Geometry check sheet. Reference: the model listing, model coordinates, mm. A direction names the side the tool comes from. Round coordinates to 2 decimals unless told otherwise and drop trailing zeros. Order: outer loops, then holes, each group sorted by start corner. A loop starts at its lowest first (then second) coordinate and runs counter-clockwise, first axis right, second up.
(1) Set-up check for faces 1 (the face through (-19, 12, 11)), 2 (the face through (34.479, 8.248, 15.287)), 3 (the face through (-19, -9, 17)): record each of +Z, -Z, +X, -X, +Y, -Y from which the full face is reachable in a straight line by a thin tool's end or side.
(2) Sectioned sample at A-A (x = -1.5). Record the boundary of the cut face in (y, z).
(3) Sectioned sample at B-B (z = 7). Give the number of separate pieces and of enclosed holes in the cut face, plus the area to 3 significant figures.
(4) Go/stop test with flat-tipped pins: pin 1 (4 mm diameter, centred on x = 29.5, y = 11.5, fed in from -Z); pin 2 (2 mm diameter, centred on x = 35, z = 12.5, fed in from -Y). Record where each tip stops, or that it passes through.
(5) Material ranges on line 1 along X through (y, z) = (15.5, 7.75); line 2 along Y through (x, z) = (2, 6.5); line 3 along X through (y, z) = (1, 4), recorded low to high.
(6) Release check for a two-part mould opening along X. For faces 4 (the face through (35.287, 17.248, 9.86)), 5 (the face through (34.479, 8.287, 9.752)), 6 (the face through (-32.1, 14.14, 7.89)) record: +X half, -X half, draft (parallel to the pull), parting line (faces both ways), or undercut.
(7) Sectioned sample at C-C (y = 14). Record the boundary of the cut face in (x, z), plus the area to 3 significant figures.
(8) Sectioned sample at D-D (z = 16.75). Record the boundary of the cut face in (x, y).
from build123d import *

# Parameters (mm, degrees)
PAD_DEPTH            = 20
POCKET_DEPTH         = 16
SKETCH002_R          = 1.75
SKETCH002_W          = 28
SKETCH002_H          = 22
POCKET001_DEPTH      = 4
POCKET002_DEPTH      = 3
SKETCH004_W          = 27
SKETCH004_H          = 18
POCKET003_DEPTH      = 3
SKETCH005_R          = 1
POCKET004_DEPTH      = 10
SKETCH007_W          = 13
SKETCH007_H          = 11
PAD001_DEPTH         = 6
POCKET005_DEPTH      = 5
POCKET005_DEPTH_BACK = 10
SKETCH008_R          = 4
POCKET006_DEPTH      = 3
SKETCH009_R          = 3.5
POCKET007_DEPTH      = 3


with BuildPart() as part:
    # Sketch001 (on Sketch) → Pad (new body)
    with BuildSketch(Plane.XY):
        with BuildLine():
            Line((-33.5, 18), (33.5, 18))
            ThreePointArc((36, 15.5), (35.267767, 17.267767), (33.5, 18))
            Line((36, 15.5), (36, -15.5))
            ThreePointArc((33.5, -18), (35.267767, -17.267767), (36, -15.5))
            Line((33.5, -18), (-33.5, -18))
            ThreePointArc((-36, -15.5), (-35.267767, -17.267767), (-33.5, -18))
            Line((-36, -15.5), (-36, 15.5))
            ThreePointArc((-33.5, 18), (-35.267767, 17.267767), (-36, 15.5))
        make_face()
    extrude(amount=PAD_DEPTH)

    # Sketch → Pocket (cut)
    with BuildSketch(Plane.XY):
        with BuildLine():
            Line((-30, 15), (30, 15))
            ThreePointArc((33, 12), (32.12132, 14.12132), (30, 15))
            Line((33, 12), (33, -12))
            ThreePointArc((30, -15), (32.12132, -14.12132), (33, -12))
            Line((30, -15), (-30, -15))
            ThreePointArc((-33, -12), (-32.12132, -14.12132), (-30, -15))
            Line((-33, -12), (-33, 12))
            ThreePointArc((-30, 15), (-32.12132, 14.12132), (-33, 12))
        make_face()
    extrude(amount=POCKET_DEPTH, mode=Mode.SUBTRACT)

    # Sketch002 (on Sketch) → Pocket001 (cut)
    with BuildSketch(Plane.XY.offset(20)):
        with Locations((-29.5, -11.5)):
            Circle(SKETCH002_R)
        with Locations((29.5, 11.5)):
            Circle(SKETCH002_R)
        with Locations((11, -2.5)):
            Rectangle(SKETCH002_W, SKETCH002_H)
    extrude(amount=-POCKET001_DEPTH, mode=Mode.SUBTRACT)

    # Sketch003 (on Face15 of Pocket001) → Pocket002 (cut)
    with BuildSketch(Plane(origin=(33, 0, 0), x_dir=(0, -1, 0), z_dir=(-1, 0, 0))):
        with BuildLine():
            Line((-6.5, 16), (-1.5, 16))
            ThreePointArc((1, 13.5), (0.267767, 15.267767), (-1.5, 16))
            Line((1, 13.5), (1, 11.5))
            ThreePointArc((-1.5, 9), (0.267767, 9.732233), (1, 11.5))
            Line((-1.5, 9), (-6.5, 9))
            ThreePointArc((-9, 11.5), (-8.267767, 9.732233), (-6.5, 9))
            Line((-9, 11.5), (-9, 13.5))
            ThreePointArc((-6.5, 16), (-8.267767, 15.267767), (-9, 13.5))
        make_face()
    extrude(amount=-POCKET002_DEPTH, mode=Mode.SUBTRACT)

    # Sketch004 (on Face33 of Pocket002) → Pocket003 (cut)
    with BuildSketch(Plane(origin=(0, 0, 16), x_dir=(1, 0, 0), z_dir=(0, 0, -1))):
        with Locations((-18.5, 0)):
            Rectangle(SKETCH004_W, SKETCH004_H)
    extrude(amount=-POCKET003_DEPTH, mode=Mode.SUBTRACT)

    # Sketch005 → Pocket004 (cut)
    with BuildSketch(Plane.XY):
        with Locations((-33.7, -15.7)):
            Circle(SKETCH005_R)
        with Locations((33.7, -15.7)):
            Circle(SKETCH005_R)
        with Locations((33.7, 15.7)):
            Circle(SKETCH005_R)
        with Locations((-33.7, 15.7)):
            Circle(SKETCH005_R)
    extrude(amount=POCKET004_DEPTH, mode=Mode.SUBTRACT)

    # Sketch007 (on Face18 of Pocket004) → Pad001 (join)
    with BuildSketch(Plane.XZ.offset(-15)):
        with Locations((-18.5, 5.5)):
            Rectangle(SKETCH007_W, SKETCH007_H)
    extrude(amount=PAD001_DEPTH)

    # Sketch006 (on Face18 of Pocket004) → Pocket005 (cut, two sides)
    with BuildSketch(Plane.XZ.offset(-15)) as pocket005_sk:
        with BuildLine():
            Line((-21, 10), (-16, 10))
            ThreePointArc((-14, 8), (-14.585786, 9.414214), (-16, 10))
            Line((-14, 8), (-14, 3))
            ThreePointArc((-16, 1), (-14.585786, 1.585786), (-14, 3))
            Line((-16, 1), (-21, 1))
            ThreePointArc((-23, 3), (-22.414214, 1.585786), (-21, 1))
            Line((-23, 3), (-23, 8))
            ThreePointArc((-21, 10), (-22.414214, 9.414214), (-23, 8))
        make_face()
    extrude(amount=-POCKET005_DEPTH, mode=Mode.SUBTRACT)
    extrude(pocket005_sk.sketch, amount=POCKET005_DEPTH_BACK, mode=Mode.SUBTRACT)

    # Sketch008 → Pocket006 (cut)
    with BuildSketch(Plane.YZ.offset(36)):
        with Locations((-7.5, 7)):
            Circle(SKETCH008_R)
    extrude(amount=-POCKET006_DEPTH, mode=Mode.SUBTRACT)

    # Sketch009 (on Face1 of Pocket006) → Pocket007 (cut)
    with BuildSketch(Plane(origin=(-36, 0, 0), x_dir=(0, -1, 0), z_dir=(-1, 0, 0))):
        with Locations((7, 0)):
            Circle(SKETCH009_R)
    extrude(amount=-POCKET007_DEPTH, mode=Mode.SUBTRACT)


solid = part.part
Answer below:
1. face 1: none
1. face 2: +X
1. face 3: -Z
2. outline: (-18, 0) - (-15, 0) - (-15, 16) - (-13.5, 16) - (-13.5, 20) - (-18, 20) - close; (8.5, 16) - (15, 16) - (15, 0) - (18, 0) - (18, 20) - (8.5, 20) - close
3. separate pieces: 2
3. enclosed holes: 4
3. area: 575 mm2
4. pin 1: stops at z = 16
4. pin 2: stops at y = -17.95
5. line 1: x = -36 to -34.68, -32.72 to -23, -14 to 32.72, 34.68 to 36
5. line 2: y = -18 to -15, 15 to 18
5. line 3: x = -36 to -33, 33 to 36
6. face 4: +X half
6. face 5: draft
6. face 6: undercut
7. outline: (-36, 0) - (-32.24, 0) - (-32.24, 16) - (32.24, 16) - (32.24, 0) - (36, 0) - (36, 20) - (-36, 20) - close; (-25, 0) - (-12, 0) - (-12, 11) - (-25, 11) - close; hole (-23, 3) arc R2 ccw to (-21, 1) - (-16, 1) arc R2 ccw to (-14, 3) - (-14, 8) arc R2 ccw to (-16, 10) - (-21, 10) arc R2 ccw to (-23, 8) - close
7. area: 474 mm2
8. outline: (-36, -15.5) arc R2.5 ccw to (-33.5, -18) - (33.5, -18) arc R2.5 ccw to (36, -15.5) - (36, 15.5) arc R2.5 ccw to (33.5, 18) - (-33.5, 18) arc R2.5 ccw to (-36, 15.5) - close; hole (-32, -9) - (-5, -9) - (-5, 9) - (-32, 9) - close; hole circle Ø3.5 at (-29.5, -11.5); hole (-3, -13.5) - (25, -13.5) - (25, 8.5) - (-3, 8.5) - close; hole circle Ø3.5 at (29.5, 11.5)
